Answer from the drawing. Dimensions are ordinates in mm from the lowest x, y and z of the part. A direction names the side the tool comes from. Give positions to 0.01 mm unless a question says otherwise; leave off trailing zeros. Write each loop counter-clockwise with the first axis right and the second up, starting at its lowest first coordinate (ties: lowest second). Pieces come first, ordered by that corner, then holes. Notation, with made-up numbers: (75, -20.75) -> (125, -20.75) arc R23 cw to (125, 6.25) -> close; hole circle Ø11 at (38, -39). An arc over 180 degrees is marked (long way). Use a Markdown table: item, result. Add a question column.
Q1. Section C-C, the plane z = 38 is taken. Give the vertices of the cut face in (x, y).
Q2. Section D-D, the plane z = 4.5 is taken. Give the vertices of the cut face in (x, y).
Q3. Section B-B, the plane y = 32 is taken. Give the vertices of the cut face in (x, z).
Q4. Consider line 1 (Y direction, x = 32, z = 40.5); line 2 (Z direction, x = 32, y = 45.45); line 3 (Z direction, x = 36.5, y = 32). Determine where each line is inside the solid, lowest interval first.
Q5. Section A-A, the plane x = 32 is taken. State how many separate pieces and enclosed holes the cut face has, plus the area to 3 significant figures.
Q6. Each of these flat-tipped pins is pushed along its axis until it touches: pin 1 Ø2 at (x, y) = (54, 56.5) entering from +Z; pin 2 Ø10 at (x, y) = (30, 31) entering from +Z; pin 3 Ø7 at (x, z) = (32, 30) entering from -Y. Where does it stop, or does it pass through?
Q7. For the marked faces 1 and 2, determine the directions among +Z, -Z, +X, -X, +Y, -Y from which every point of the face is accessible in a straight line to the end or side of a thin tool.
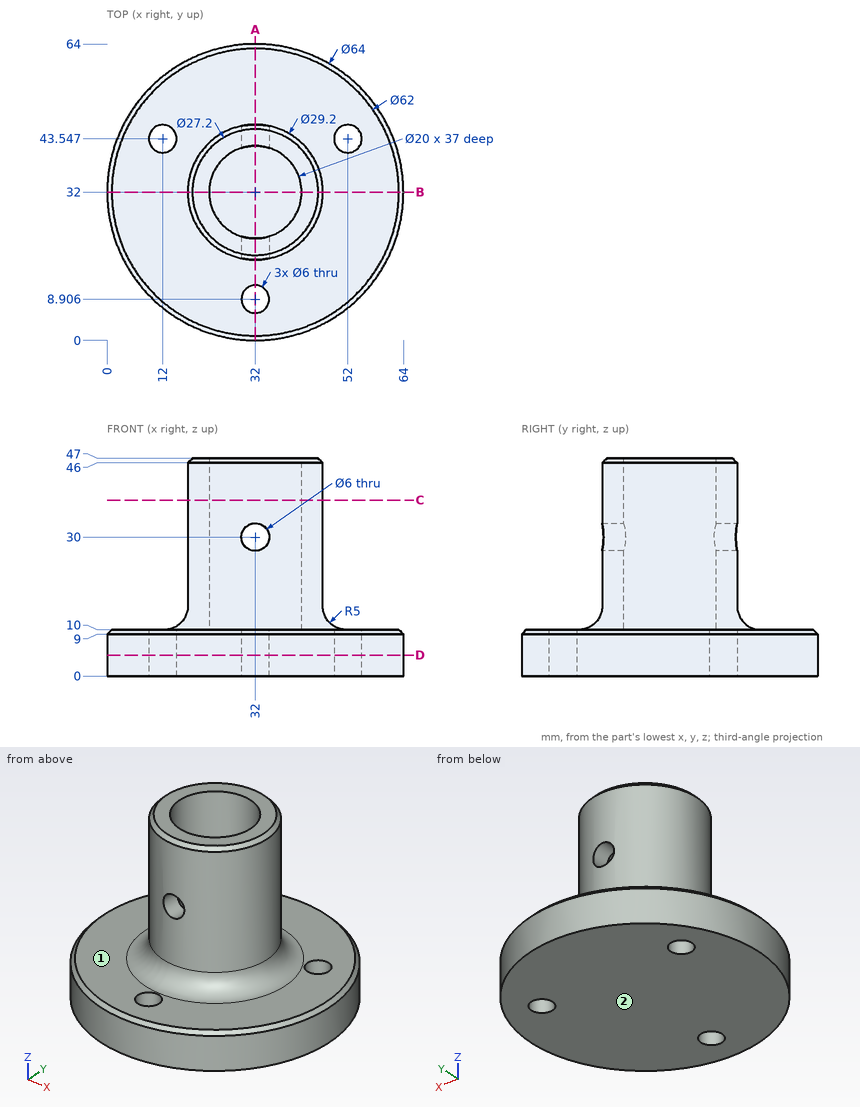
Result set:
| question | item | result |
|---|---|---|
| 1 | outline | circle Ø29.2 at (32, 32); hole circle Ø20 at (32, 32) |
| 2 | outline | circle Ø64 at (32, 32); hole circle Ø6 at (12, 43.55); hole circle Ø6 at (32, 8.91); hole circle Ø6 at (52, 43.55) |
| 3 | outline | (0, 0) -> (64, 0) -> (64, 9) -> (63, 10) -> (51.6, 10) arc R5 cw to (46.6, 15) -> (46.6, 46) -> (45.6, 47) -> (42, 47) -> (42, 10) -> (22, 10) -> (22, 47) -> (18.4, 47) -> (17.4, 46) -> (17.4, 15) arc R5 cw to (12.4, 10) -> (1, 10) -> (0, 9) -> close |
| 4 | line 1 | y = 17.4 to 22, 42 to 46.6 |
| 4 | line 2 | z = 0 to 27, 33 to 47 |
| 4 | line 3 | z = 0 to 10 |
| 5 | separate pieces | 4 |
| 5 | enclosed holes | 0 |
| 5 | area | 874 mm2 |
| 6 | pin 1 | stops at z = 9.07 |
| 6 | pin 2 | stops at z = 10 |
| 6 | pin 3 | stops at y = 17.4 |
| 7 | face 1 | +Z |
| 7 | face 2 | -Z, +X, -X, +Y, -Y |
